Geometry: see drawing. Coordinates: mm, zero at the bounding-box minimum. A direction names the side the tool comes from. Give positions to 0.01 mm unless a question says otherwise; leave off trailing zeros. Loops run counter-clockwise (first coordinate to the right, second up) from the corner with the lowest first, then second, coordinate; pieces in that order, holes last. Notation, with made-up numbers: M -37.5,72 L 11.5,72 A18 cw 11.5,92 Z; hole C -4.5,86.25 d6. An arc over 180 degrees is marked long. Put each result on its own line as item: value.
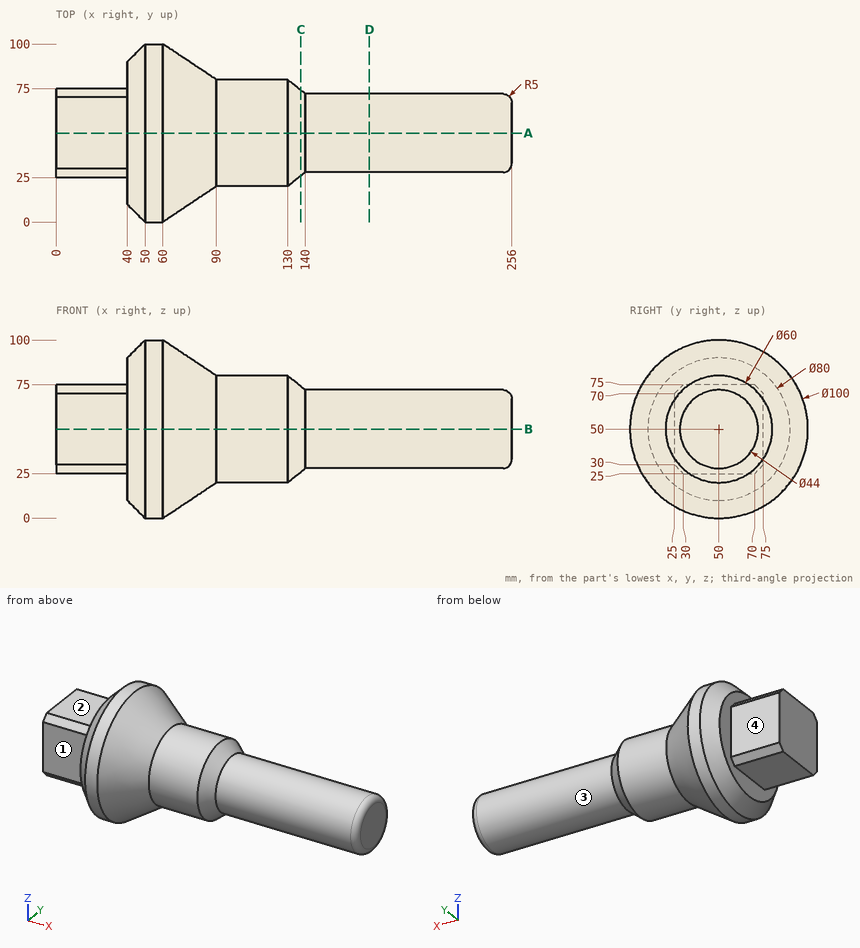
1. Material intervals for line 1 (Z direction, x = 87, y = 30); line 2 (Z direction, x = 155.5, y = 36); line 3 (Y direction, x = 19.5, z = 38), sorted ascending. Write a range as from..to.
Found:
line 1: 25.02..74.98
line 2: 33.03..66.97
line 3: 25..75
2. Access query for the marked faces 1, 2, 3 and 4. Directions: +Z, -Z, +X, -X, +Y, -Y. A direction counts if a zero-diameter tool reaches every point of the face in a straight line with its end or side. Return the directions, or none.
Found:
face 1: +Z, -Z, -X, -Y
face 2: +Z, -X, +Y, -Y
face 3: +X
face 4: +Z, -Z, -X, +Y
3. Contact query for flat-ended pins moving along their axis: P1, Ø20, axis at x = 25.5, y = 50.5, coming from the -Z side; P2, Ø10, axis at x = 42.5, z = 79.5, coming from the +Y side; P3, Ø6, axis at x = 191.5, z = 51, coming from the -Y side. Output: stop coordinate, or through.
Found:
P1: z = 25
P2: y = 88.26
P3: y = 28
4. Section query A-A (y = 50). Output: boundary loops of the cut face in (x, z).
Found:
outline: M 0,25 L 40,25 L 40,10 L 50,0 L 60,0 L 90,20 L 130,20 L 140,28 L 251,28 A5 ccw 256,33 L 256,67 A5 ccw 251,72 L 140,72 L 130,80 L 90,80 L 60,100 L 50,100 L 40,90 L 40,75 L 0,75 Z
5. Section query C-C (x = 137.5). Output: boundary loops of the cut face in (y, z).
Found:
outline: C 50,50 d48
6. Section query D-D (x = 176). Output: boundary loops of the cut face in (y, z).
Found:
outline: C 50,50 d44
